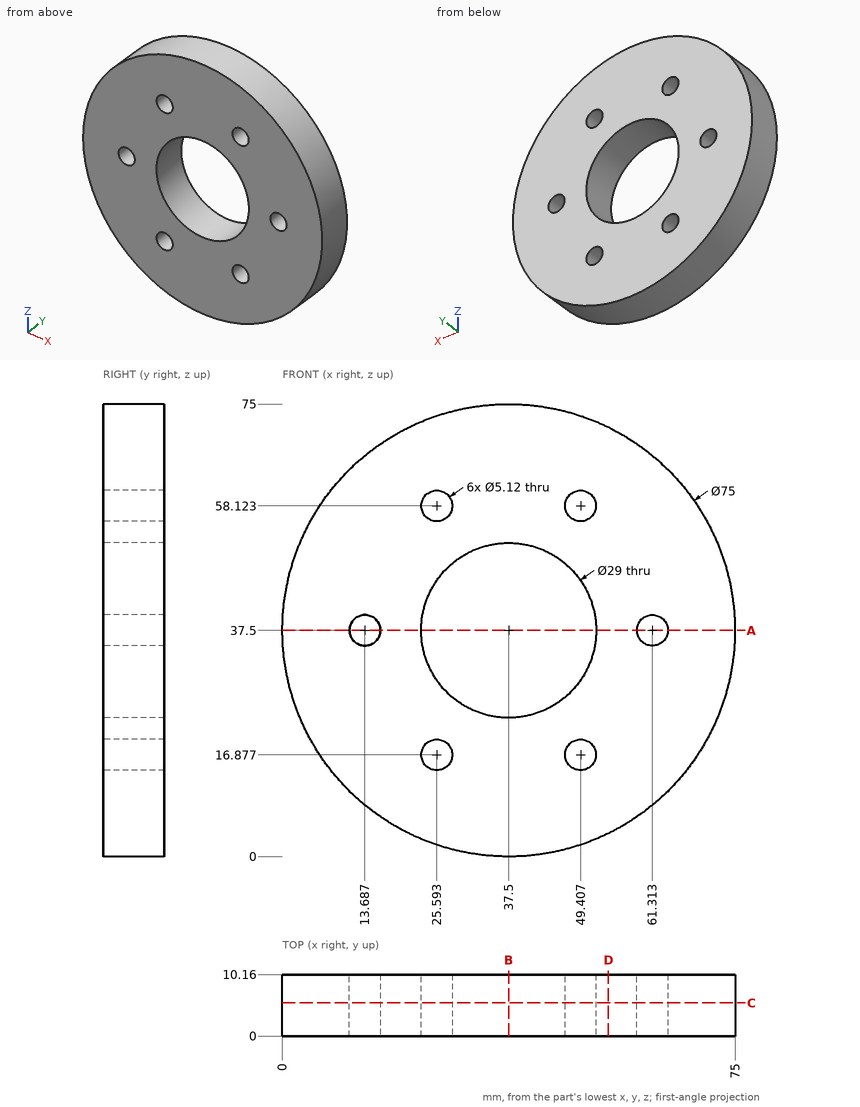
Here's the drawing with two shaded views (mm, measured from the low corner). I have some questions. Coordinates: 2 decimals unless noted, no trailing zeros. Write each loop counter-clockwise with the first axis right and the second up, starting at its lowest first coordinate (ties: lowest second). Pieces come first, ordered by that corner, then holes. Notation, with made-up numbers: (-35.5, 78) -> (-8.5, 78) arc R22 ccw to (-8.5, 89) -> close; hole circle Ø10 at (7.5, 71). An arc over 180 degrees is marked (long way). One line per question, with ' | ' between items. Start each with the question number.
1. If we section it at D-D (x = 54): Please give me the cut outline in (y, z) (1 decimal), and give its area (3 significant figures).
2. If we section it at A-A (z = 37.5): Please give me the cut outline in (x, y), and give its area (3 significant figures).
3. If we section it at C-C (y = 5.5): Please give me the cut outline in (x, z), and give its area (3 significant figures).
4. Will these pins go through, and if not, where does the flat tip stop? P1, Ø1.5, axis at y = 1.5, z = 38.5, coming from the +X side; P2, Ø6, axis at x = 54, y = 6.5, coming from the -Z side (1 decimal); P3, Ø2, axis at x = 62, y = 1.5, coming from the -Z side (1 decimal); P4, Ø4, axis at x = 25.59, z = 16.88, coming from the -Y side.
5. Please list where these lines run through material, in increasing order: line 1 along Z through (x, y) = (37, 8.75); line 2 along Z through (x, y) = (61, 7) (1 decimal); line 3 along X through (y, z) = (8, 44.5).
6. If we section it at B-B (x = 37.5): Please give me the cut outline in (y, z), and give its area (3 significant figures).
Return value:
1) outline: (0, 3.8) -> (10.2, 3.8) -> (10.2, 71.2) -> (0, 71.2) -> close | area: 684 mm²
2) outline: (0, 0) -> (11.13, 0) -> (11.13, 10.16) -> (0, 10.16) -> close; (16.25, 0) -> (23, 0) -> (23, 10.16) -> (16.25, 10.16) -> close; (52, 0) -> (58.75, 0) -> (58.75, 10.16) -> (52, 10.16) -> close; (63.87, 0) -> (75, 0) -> (75, 10.16) -> (63.87, 10.16) -> close | area: 363 mm²
3) outline: circle Ø75 at (37.5, 37.5); hole circle Ø5.12 at (13.69, 37.5); hole circle Ø29 at (37.5, 37.5); hole circle Ø5.12 at (25.59, 16.88); hole circle Ø5.12 at (25.59, 58.12); hole circle Ø5.12 at (49.41, 16.88); hole circle Ø5.12 at (49.41, 58.12); hole circle Ø5.12 at (61.31, 37.5) | area: 3,630 mm²
4) P1: stops at x = 75 | P2: stops at z = 2.5 | P3: stops at z = 8.3 | P4: passes through
5) line 1: z = 0 to 23.01, 51.99 to 75 | line 2: z = 8.3 to 35, 40 to 66.7 | line 3: x = 0.66 to 24.8, 50.2 to 74.34
6) outline: (0, 0) -> (10.16, 0) -> (10.16, 23) -> (0, 23) -> close; (0, 52) -> (10.16, 52) -> (10.16, 75) -> (0, 75) -> close | area: 467 mm²
